Source: three-view drawing plus pictorial views. Frame: mm from the lowest corner of the part. A direction names the side the tool comes from. Give positions to 0.01 mm unless a question says otherwise; leave off trailing zeros. Order: outer loops, then holes, each group sorted by start corner. A loop starts at its lowest first (then second) coordinate and runs counter-clockwise, first axis right, second up. Notation, with made-up numbers: (34, -26) -> (67, -26) arc R22 cw to (67, 2) -> close; hole circle Ø3 at (-31, 9.5). An arc over 180 degrees is marked (long way). Use a Markdown table: item, result. Add a question column.
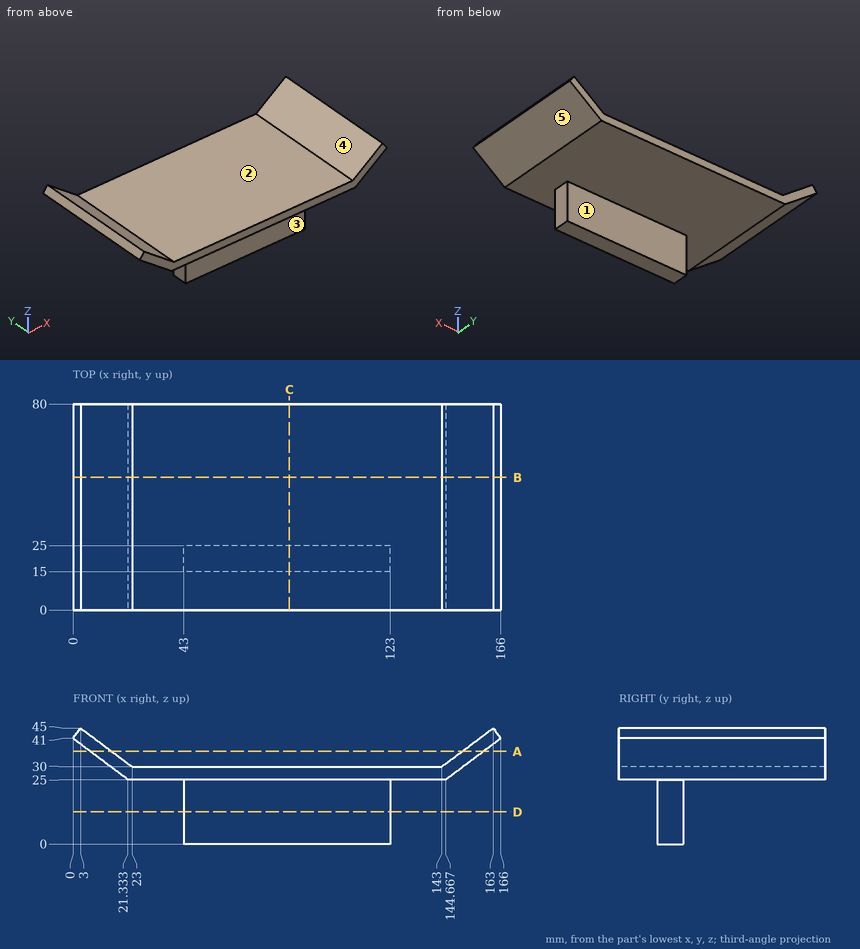
Q1. Section query C-C (x = 84). Return loops of the section in (y, z), plus the area to 3 significant figures.
Q2. First-contact query: pin 1 (1.5 mm diameter, centred on y = 25.5, z = 32.5, fed in from +X) (1 decimal); pin 2 (8 mm diameter, centred on x = 134, y = 11, fed in from +Z); pin 3 (12.5 mm diameter, centred on x = 79.5, z = 17.5, fed in from -Y). Flat tips, straight axial feed; report the tip coordinate or a pass-through.
Q3. Section query B-B (y = 51.5). Return loops of the section in (x, z).
Q4. Access query for the marked faces 1 and 2. Directions: +Z, -Z, +X, -X, +Y, -Y. A direction counts if a zero-diameter tool reaches every point of the face in a straight line with its end or side. Return the directions, or none.
Q5. Section query A-A (z = 36). Return loops of the section in (x, y).
Q6. Draft query along X for the marked faces 3, 4 and 5. Return one class per face: +X half, -X half, draft (parallel to the pull), parting line (faces both ways), or undercut.
Q7. Section query D-D (z = 12.5). Return loops of the section in (x, y).
Q8. Ray query, line 1 (Z direction, x = 32, y = 30); line 2 (Y direction, x = 52, z = 13); line 3 (Z direction, x = 44.5, y = 18.5). Return the intervals inside material, ascending.
Solution:
| question | item | result |
|---|---|---|
| 1 | outline | (0, 25) -> (15, 25) -> (15, 0) -> (25, 0) -> (25, 25) -> (80, 25) -> (80, 30) -> (0, 30) -> close |
| 1 | area | 650 mm² |
| 2 | pin 1 | stops at x = 155.7 |
| 2 | pin 2 | stops at z = 30 |
| 2 | pin 3 | stops at y = 15 |
| 3 | outline | (0, 41) -> (21.33, 25) -> (144.67, 25) -> (166, 41) -> (163, 45) -> (143, 30) -> (23, 30) -> (3, 45) -> close |
| 4 | face 1 | -Z, +X, -X, +Y |
| 4 | face 2 | +Z, +Y, -Y |
| 5 | outline | (6.67, 0) -> (15, 0) -> (15, 80) -> (6.67, 80) -> close; (151, 0) -> (159.33, 0) -> (159.33, 80) -> (151, 80) -> close |
| 6 | face 3 | draft |
| 6 | face 4 | undercut |
| 6 | face 5 | +X half |
| 7 | outline | (43, 15) -> (123, 15) -> (123, 25) -> (43, 25) -> close |
| 8 | line 1 | z = 25 to 30 |
| 8 | line 2 | y = 15 to 25 |
| 8 | line 3 | z = 0 to 30 |
